```python
from build123d import *

# Parameters (mm, degrees)
SALIENTE_EXTRUIR2_DEPTH = 30
CROQUIS3_W              = 60.629420227
CROQUIS3_H              = 60.965705304
CORTAR_EXTRUIR1_DEPTH   = 30
CROQUIS4_R              = 3
CORTAR_EXTRUIR2_DEPTH   = 54.545510937
CROQUIS5_W              = 28.284271248
CROQUIS5_H              = 30
SALIENTE_EXTRUIR3_DEPTH = 14.142136
SALIENTE_EXTRUIR4_DEPTH = 10
CROQUIS7_W              = 23.581736244
CROQUIS7_H              = 30.206171788
CORTAR_EXTRUIR3_DEPTH   = 60
CROQUIS8_R              = 3
CORTAR_EXTRUIR4_DEPTH   = 71.616578937
CROQUIS10_W             = 79.072347139
CROQUIS10_H             = 56.401254602
CORTAR_EXTRUIR5_DEPTH   = 50
CROQUIS12_W             = 30
CROQUIS12_H             = 20
SALIENTE_EXTRUIR6_DEPTH = 20
CROQUIS13_R             = 1.5
CORTAR_EXTRUIR6_DEPTH   = 20


with BuildPart() as part:
    # Croquis2 → Saliente-Extruir2 (new body)
    with BuildSketch(Plane(origin=(0, 0, 0), x_dir=(0, 0, -1), z_dir=(1, 0, 0))):
        Polygon((0, 0), (-50, 0), (-75.724787771, -15.434872663), (-75.724787771, -45.434872663), (-55.724787771, -45.434872663), (-55.724787771, -26.758680242), (-44.460320701, -20), (0, -20), align=None)
    extrude(amount=SALIENTE_EXTRUIR2_DEPTH)

    # Croquis3 → Cortar-Extruir1 (cut)
    with BuildSketch(Plane(origin=(-22.862393886, 0, 22.862393886), x_dir=(0.707106781, 0, 0.707106781), z_dir=(-0.707106781, 0, 0.707106781))):
        with Locations((51.516510193, -19.86952732)):
            Rectangle(CROQUIS3_W, CROQUIS3_H)
    extrude(amount=CORTAR_EXTRUIR1_DEPTH, mode=Mode.SUBTRACT)

    # Croquis4 → Cortar-Extruir2 (cut, through all)
    with BuildSketch(Plane(origin=(-22.862393886, 0, 22.862393886), x_dir=(0.707106781, 0, 0.707106781), z_dir=(-0.707106781, 0, 0.707106781))):
        with Locations((60.616578749, -34.226076292)):
            Circle(CROQUIS4_R)
    extrude(amount=-CORTAR_EXTRUIR2_DEPTH, mode=Mode.SUBTRACT)

    # Croquis5 → Saliente-Extruir3 (add)
    with BuildSketch(Plane(origin=(-22.862393886, 0, 22.862393886), x_dir=(0.707106781, 0, 0.707106781), z_dir=(-0.707106781, 0, 0.707106781))):
        with Locations((60.616578749, -30.434872663)):
            Rectangle(CROQUIS5_W, CROQUIS5_H)
    extrude(amount=-SALIENTE_EXTRUIR3_DEPTH)

    # Croquis6 → Saliente-Extruir4 (add)
    with BuildSketch(Plane(origin=(-22.862393886, 0, 22.862393886), x_dir=(0.707106781, 0, 0.707106781), z_dir=(-0.707106781, 0, 0.707106781))):
        Polygon((32.332307501, -20.758680242), (46.474443125, -26.758680242), (46.474443125, -45.434872663), (74.758714373, -45.434872663), (74.758714373, -15.434872663), (38.378370617, 0), (32.332307501, 0), align=None)
    extrude(amount=SALIENTE_EXTRUIR4_DEPTH)

    # Croquis7 → Cortar-Extruir3 (cut)
    with BuildSketch(Plane(origin=(0, 0, 0), x_dir=(1, 0, 0), z_dir=(0, 1, 0))):
        with Locations((-11.790868122, -58.05803285)):
            Rectangle(CROQUIS7_W, CROQUIS7_H)
    extrude(amount=-CORTAR_EXTRUIR3_DEPTH, mode=Mode.SUBTRACT)

    # Croquis8 → Cortar-Extruir4 (cut, through all)
    with BuildSketch(Plane(origin=(-29.933461698, 0, 29.933461698), x_dir=(0.707106781, 0, 0.707106781), z_dir=(-0.707106781, 0, 0.707106781))):
        with Locations((60.616578749, -35.434872663)):
            Circle(CROQUIS8_R)
    extrude(amount=-CORTAR_EXTRUIR4_DEPTH, mode=Mode.SUBTRACT)

    # Croquis10 → Cortar-Extruir5 (cut)
    with BuildSketch(Plane(origin=(0, 22.058823529, 13.235294118), x_dir=(1, 0, 0), z_dir=(0, 0.857492926, 0.514495755))):
        with Locations((7.523719949, -68.590647859)):
            Rectangle(CROQUIS10_W, CROQUIS10_H)
    extrude(amount=CORTAR_EXTRUIR5_DEPTH, mode=Mode.SUBTRACT)

    # Croquis12 → Saliente-Extruir6 (add)
    with BuildSketch(Plane(origin=(0, 0, 0), x_dir=(-1, 0, 0), z_dir=(0, 0, -1))):
        with Locations((-15, -10)):
            Rectangle(CROQUIS12_W, CROQUIS12_H)
    extrude(amount=SALIENTE_EXTRUIR6_DEPTH)

    # Croquis13 → Cortar-Extruir6 (cut)
    with BuildSketch(Plane.XZ.offset(20)):
        with Locations((15, -10)):
            Circle(CROQUIS13_R)
        with Locations((15, 10)):
            Circle(CROQUIS13_R)
    extrude(amount=-CORTAR_EXTRUIR6_DEPTH, mode=Mode.SUBTRACT)


solid = part.part
```
The listing builds one solid part. Answer for the finished solid, in the listing's coordinates (mm). A direction names the side the tool comes from. Coordinates: 2 decimals unless noted, no trailing zeros. Order: outer loops, then holes, each group sorted by start corner. A loop starts at its lowest first (then second) coordinate and runs counter-clockwise, first axis right, second up. Notation, with made-up numbers: M 46,40.25 L 62,40.25 A15 cw 62,48.25 Z; hole C -0.5,-15 d1. An arc over 180 degrees is marked long. Answer as a JSON object with one key per item and string values. Group by question number.
1. Section B-B on y = -34 is taken. Write down the section's boundary in (x, z), then the cut area to 3 significant figures.
2. Flat-ended cylindrical pins translate along their axes: P1, Ø3, axis at x = 29.5, y = -36.5, coming from the -Z side; P2, Ø21.5, axis at y = -7, z = 25, coming from the +X side; P3, Ø5, axis at x = 35.5, z = 69, coming from the +Y side; P4, Ø2.5, axis at x = 15, z = -10, coming from the +Y side. Find the tip coordinate at first contact, or state that the pin passes through.
3. Determine the mould class of faces 6 (the flat face through (15, 0, 15)), 7 (the flat face through (21, -45.435, 64)), 8 (the cylindrical face through (20.885, -38.364, 63.92)) for opening direction Y: released by +Y, released by -Y, zero draft, split by the parting line, or undercut.
4. Section A-A on z = -10 is taken. Write down the section's boundary in (x, y), then the cut area to 3 significant figures.
5. A tool of negligible diameter and unlimited length cuts with its end or side. For faces 1 (the flat face through (15, -20, 13)), 2 (the flat face through (11.584, -35.666, 54.141)), 3 (the flat face through (29.86, -30.225, 55.585)), 4 (the flat face through (34, -15.435, 66)), 5 (the flat face through (14.79, -21.925, 47.668)), from which of +Z, -Z, +X, -X, +Y, -Y can it reach the whole face along a straight path? Write none if from no direction.
6. Section C-C on y = -13 is taken. Write down the section's boundary in (x, z), then the cut area to 3 significant figures.
7. Straight lines are drawn through the part: line 1 (Z direction, x = 15, y = -3.75); line 2 (Z direction, x = 15, y = -10); line 3 (Y direction, x = 34, z = 62). For each, find the intervals that lie inside material, in ascending order.
8. Section D-D on z = 25 is taken. Write down the section's boundary in (x, y), then the cut area to 3 significant figures.
Values follow:
{
 "1": {"outline": "M 2.93,62.8 L 20,45.72 L 28.14,53.86 L 11.07,70.93 Z; M 14.79,74.66 L 31.86,57.59 L 40,65.72 L 22.93,82.8 Z", "area": "556 mm2"},
 "2": {"P1": "z = 53.72", "P2": "x = 30", "P3": "y = -15.43", "P4": "through"},
 "3": {"face 6": "released by +Y", "face 7": "released by -Y", "face 8": "undercut"},
 "4": {"outline": "M 0,-20 L 13.5,-20 L 13.5,0 L 0,0 Z; M 16.5,-20 L 30,-20 L 30,0 L 16.5,0 Z", "area": "540 mm2"},
 "5": {"face 1": "-Z, +X, -X, -Y", "face 2": "-Z, -X, -Y", "face 3": "-Z, +X, -Y", "face 4": "+Z, -Z, +X, +Y", "face 5": "-Z, -Y"},
 "6": {"outline": "M 0,-20 L 30,-20 L 30,71.67 L 11.8,71.67 L 0,59.87 Z; hole C 15,-10 d3; hole C 15,10 d3", "area": "2,670 mm2"},
 "7": {"line 1": "-20 to -11.5, -8.5 to 8.5, 11.5 to 56.25", "line 2": "-20 to -11.5, -8.5 to 8.5, 11.5 to 66.67", "line 3": "-45.43 to -15.43"},
 "8": {"outline": "M 0,-20 L 30,-20 L 30,0 L 0,0 Z", "area": "600 mm2"}
}
